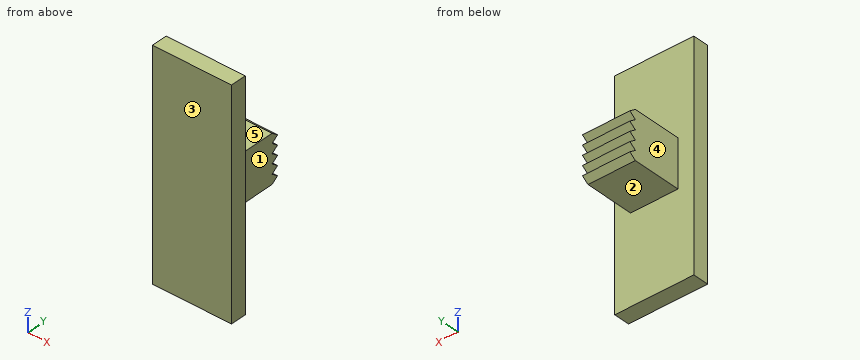
```python
from build123d import *

# Parameters (mm, degrees)
BOSS_EXTRU_1_DEPTH      = 1.5
BOSS_EXTRU_1_DEPTH_BACK = 1.5
ESQUISSE2_W             = 14
ESQUISSE2_H             = 1
BOSS_EXTRU_2_DEPTH      = 1


with BuildPart() as part:
    # Esquisse1 → Boss.-Extru.1 (new, two sides: drawn at the far end of the back side and taken through both)
    with BuildSketch(Plane(origin=(0, 0, 0), x_dir=(0, 0, -1), z_dir=(1, 0, 0)).offset(-BOSS_EXTRU_1_DEPTH_BACK)):
        Polygon((-7, 0), (-1.5, 0), (-1.5, 3.1), (-1.2, 3.5), (-0.9, 3.1), (-0.6, 3.5), (-0.3, 3.1), (0, 3.5), (0.3, 3.1), (0.6, 3.5), (0.9, 3.1), (1.2, 3.5), (1.5, 3.1), (1.5, 0), (7, 0), (7, -1), (-7, -1), align=None)
    extrude(amount=BOSS_EXTRU_1_DEPTH + BOSS_EXTRU_1_DEPTH_BACK)

    # Esquisse2 → Boss.-Extru.2 (add)
    with BuildSketch(Plane(origin=(1.5, 0, 0), x_dir=(0, 0, -1), z_dir=(1, 0, 0))):
        with Locations((0, -0.5)):
            Rectangle(ESQUISSE2_W, ESQUISSE2_H)
    boss_extru_2 = extrude(amount=BOSS_EXTRU_2_DEPTH)

    # Symétrie1: Boss.-Extru.2 across plane
    add(boss_extru_2.mirror(Plane(origin=(0, 0, 0), x_dir=(0, 0, 1), z_dir=(1, 0, 0))))


solid = part.part
```
Here's how the part is built. I have some questions about the finished solid (model axes, mm). Face numbers are marked on the shaded views. A direction names the side the tool comes from. Round coordinates to 2 decimals unless told otherwise and drop trailing zeros. Write each loop counter-clockwise with the first axis right and the second up, starting at its lowest first coordinate (ties: lowest second). Pieces come first, ordered by that corner, then holes.
Q1. If we section it at A-A on x = 0.6: Write out the boundary of the cut face in (y, z), plus the area to 3 significant figures.
Q2. If we section it at D-D on z = -2.75: Write out the boundary of the cut face in (x, y), plus the area to 3 significant figures.
Q3. If we section it at C-C on y = 1.25: Write out the boundary of the cut face in (x, z).
Q4. Please list where these lines run through material, in increasing order: probe 1 along Y at (x, z) = (-1.75, 2.25); probe 2 along Z at (x, y) = (0.4, 3).
Q5. Will these pins go through, and if not, where does the flat tip stop? P1, Ø2.5, axis at y = 1.5, z = 0, coming from the +X side; P2, Ø2, axis at x = -1.5, y = 3, coming from the -Z side; P3, Ø1.5, axis at x = 0.5, z = -1.5, coming from the +Y side.
Q6. Which directions (+Z, -Z, +X, -X, +Y, -Y) give clear straight access to the entire face, cutting with the end or side of a thin tool? Please do the marked faces 1, 2, 3, 4 and 5.
Q7. If we section it at B-B on z = -0.75: Write out the boundary of the cut face in (x, y).
Answer below:
1. outline: (-1, -7) - (0, -7) - (0, -1.5) - (3.1, -1.5) - (3.5, -1.2) - (3.1, -0.9) - (3.5, -0.6) - (3.1, -0.3) - (3.5, 0) - (3.1, 0.3) - (3.5, 0.6) - (3.1, 0.9) - (3.5, 1.2) - (3.1, 1.5) - (0, 1.5) - (0, 7) - (-1, 7) - close
1. area: 23.9 mm2
2. outline: (-2.5, -1) - (2.5, -1) - (2.5, 0) - (-2.5, 0) - close
2. area: 5.00 mm2
3. outline: (-1.5, -1.5) - (1.5, -1.5) - (1.5, 1.5) - (-1.5, 1.5) - close
4. probe 1: y = -1 to 0
4. probe 2: z = -1.5 to 1.5
5. P1: stops at x = 1.5
5. P2: stops at z = -1.5
5. P3: stops at y = 3.5
6. face 1: +Z, -Z, +X, +Y
6. face 2: -Z, +X, -X, +Y
6. face 3: +Z, -Z, +X, -X, -Y
6. face 4: +Z, -Z, -X, +Y
6. face 5: +Z, +X, -X, +Y
7. outline: (-2.5, -1) - (2.5, -1) - (2.5, 0) - (1.5, 0) - (1.5, 3.3) - (-1.5, 3.3) - (-1.5, 0) - (-2.5, 0) - close
